The listing builds one solid part. Answer for the finished solid, in the listing's coordinates (mm). A direction names the side the tool comes from. Give positions to 0.01 mm unless a question says otherwise; leave off trailing zeros. Write each loop counter-clockwise with the first axis right and the second up, starting at its lowest first coordinate (ties: lowest second). Pieces come first, ordered by that corner, then holes. Notation, with made-up numbers: M 87,25 L 129,25 A9 cw 129,32 Z; hole C -14.5,-18 d4. An arc over 180 degrees is marked long. Answer as a JSON object with one key per item and string values.
Autodesk Inventor part; units mm, degrees
ref_plane "YZ Plane" through (0, 0, 0) normal (1, 0, 0) x (0, 1, 0)
ref_plane "XZ Plane" through (0, 0, 0) normal (0, 1, 0) x (-1, 0, 0)
ref_plane "XY Plane" through (0, 0, 0) normal (0, 0, 1) x (1, 0, 0)
sketch "Sketch1" plane through (0, 0, 0) normal (0, 0, 1) x (1, 0, 0)
  line L0 (-17.6048, 17.9341) -> (10.9702, 17.9341)
  line L1 (10.9702, 17.9341) -> (10.9702, -64.9334)
  line L2 (10.9702, -64.9334) -> (-17.6048, -64.9334)
  line L3 (-17.6048, -64.9334) -> (-17.6048, 17.9341)
  circle A0 centre (-3.3173, 17.9341) radius 14.2875
  point P0 (0, 0)
  dimension "d0" = 28.575
  dimension "d1" = 82.8675
revolve "Revolution1" add sketch "Sketch1" angle 360 about axis through (10.9702, -64.9334, 0) along (-1, 0, 0)
sketch "Sketch2" plane through (10.9702, -64.9334, 0) normal (1, 0, 0) x (0, 0, -1)
  circle A0 centre (0, 0) radius 82.8675
  circle A1 centre (0, 0) radius 23.8125
  circle A2 centre (0, 0) radius 12.7
  line L0 (0, 0) -> (0, 42.8884)
  line L1 (37.1175, 21.4298) -> (0, 0)
  line L2 (0, 0) -> (31.3254, -18.0857)
  line L3 (31.3254, -18.0857) -> (0, 0)
  line L4 (0, 0) -> (0, -34.1508)
  line L5 (0, -34.1508) -> (0, 0)
  line L6 (0, 0) -> (-30.532, -17.6277)
  line L7 (-30.532, -17.6277) -> (0, 0)
  line L8 (0, 0) -> (-29.5082, 17.0365)
  circle A3 centre (0, 0) radius 14.2875
  point P0 (0, 64.9334)
  point P1 (0, 23.8125)
  point P2 (20.6222, 11.9063)
  point P3 (20.6222, -11.9062)
  point P4 (0, -23.8125)
  point P5 (-20.6222, -11.9063)
  point P6 (-20.6222, 11.9062)
  dimension "d3" = 47.625
  dimension "d4" = 25.4
  dimension "d5" = 60
  dimension "d6" = 60
  dimension "d7" = 60
  dimension "d8" = 60
  dimension "d16" = 28.575
hole "Hole1" at (10.9702, -41.1209, 0) at (10.9702, -53.0271, -20.6222) at (10.9702, -76.8396, -20.6222) at (10.9702, -88.7459, 0) at (10.9702, -76.8396, 20.6222) at (10.9702, -53.0271, 20.6222) direction (-1, 0, 0) diameter 5.08 depth 50.8 tip angle 118
extrude "Extrusion1" cut sketch "Sketch2" against normal blind 50.8 contours L1 L0 A2 | A2 L2 L1 | A2 L4 L2 | L0 L8 A2 | L4 A2 L6 | L6 A2 L8
extrude "Extrusion2" cut sketch "Sketch2" against normal blind 9.525 contours A3 L2 A2 L1 | L1 A2 L0 A3 | A3 L4 A2 L2 | L0 A2 L8 A3 | A3 L6 A2 L4 | L8 A2 L6 A3
sketch "Sketch3" plane through (-17.6048, -64.9334, 0) normal (-1, 0, 0) x (0, 0, 1)
  circle A0 centre (0, 0) radius 12.7
  circle A1 centre (0, 0) radius 82.8675
  circle A2 centre (0, 0) radius 14.2875
  point P0 (0, 64.9334)
  dimension "d21" = 28.575
extrude "Extrusion3" cut sketch "Sketch3" against normal blind 9.525 contours A2
properties part number "pneumatic 8'' wheel sketchy quality"
1. For faces 3 (the flat face through (1.445, -66, 13)), 4 (the cylindrical face through (-3.517, -54.744, -18.75)), 5 (the cylindrical face through (-12.91, -78.88, -3.1)), determine the directions among +Z, -Z, +X, -X, +Y, -Y from which every point of the face is accessible in a straight line to the end or side of a thin tool.
Verdict:
{"face 3": "+X", "face 4": "+X, -X", "face 5": "-X"}
2. Flat-ended cylindrical pins translate along their axes: pin 1 (4 mm diameter, centred on x = -14, y = -65.5, fed in from -Z); pin 2 (3 mm diameter, centred on x = -14, y = -95.5, fed in from -Z); pin 3 (10 mm diameter, centred on x = -1.5, z = -61, fed in from -Y). Find the tip coordinate at first contact, or state that the pin passes through.
Verdict:
{"pin 1": "stops at z = -94.21", "pin 2": "stops at z = -88.79", "pin 3": "stops at y = -144.24"}
3. A cutting plane is placed at C-C, the plane x = -14. Give the vertices of the cut face in (y, z) (1 decimal), plus the area to 3 significant figures.
Verdict:
{"outline": "C -64.9,0 d184.7; hole C -88.7,0 d5.1; hole C -76.8,-20.6 d5.1; hole C -76.8,20.6 d5.1; hole C -64.9,0 d28.6; hole C -53,-20.6 d5.1; hole C -53,20.6 d5.1; hole C -41.1,0 d5.1", "area": "26,000 mm2"}
4. The mould has two halves that part along Z. Classify faces 1 (the flat face through (-17.605, -66, 17)), 2 (the cylindrical face through (-3.517, -91.264, 0.331)): released by +Z, released by -Z, zero draft, split by the parting line, or undercut.
Verdict:
{"face 1": "zero draft", "face 2": "undercut"}
5. A cutting plane is placed at A-A, the plane z = 0. Give the vertices of the cut face in (x, y) (1 decimal), plus the area to 3 significant figures.
Verdict:
{"outline": "M -17.6,-147.8 A14.3 ccw 11,-147.8 L 11,-91.3 L -17.6,-91.3 Z; M -17.6,-86.2 L 11,-86.2 L 11,-79.2 L 1.4,-79.2 L 1.4,-77.6 L -8.1,-77.6 L -8.1,-79.2 L -17.6,-79.2 Z; M -17.6,-50.6 L -8.1,-50.6 L -8.1,-52.2 L 1.4,-52.2 L 1.4,-50.6 L 11,-50.6 L 11,-43.7 L -17.6,-43.7 Z; M -17.6,-38.6 L 11,-38.6 L 11,17.9 A14.3 ccw -17.6,17.9 Z", "area": "4,300 mm2"}
6. A cutting plane is placed at B-B, the plane x = 8.75. Give the vertices of the cut face in (y, z) (1 decimal).
Verdict:
{"outline": "C -64.9,0 d181; hole C -88.7,0 d5.1; hole C -76.8,-20.6 d5.1; hole C -76.8,20.6 d5.1; hole C -64.9,0 d28.6; hole C -53,-20.6 d5.1; hole C -53,20.6 d5.1; hole C -41.1,0 d5.1"}
7. Consider line 1 along Y through (x, z) = (-2.25, 0); line 2 along Y through (x, z) = (-3.25, 0); line 3 along Y through (x, z) = (9, 22.5). Determine where each line is inside the solid, lowest interval first.
Verdict:
{"line 1": "y = -162.05 to -91.29, -86.21 to -77.63, -52.23 to -43.66, -38.58 to 32.18", "line 2": "y = -162.09 to -91.29, -86.21 to -77.63, -52.23 to -43.66, -38.58 to 32.22", "line 3": "y = -152.19 to -78.55, -75.13 to -54.74, -51.32 to 22.32"}
